```python
from build123d import *

# Parameters (mm, degrees)
SKETCH4_R          = 0.5
CUT_EXTRUDE1_DEPTH = 24.108440155
SKETCH5_R          = 2.5
CUT_EXTRUDE2_DEPTH = 2


with BuildPart() as part:
    # Loft1: read off the stored shape, not the designer's step
    # Loft1: loft between two sections, ruled curve by curve
    loft1_from = [
        Edge.make_bspline([(4.934796286, 0, 0.8048513), (3.325093686, 0, 10.674443872), (-6.544498886, 0, 9.064741272), (-4.934796286, 0, -0.8048513), (-3.325093686, 0, -10.674443872), (6.544498886, 0, -9.064741272), (4.934796286, 0, 0.8048513)], [0, 0, 0, 0, 0.5, 0.5, 0.5, 1, 1, 1, 1], 3, [1, 0.333333333, 0.333333333, 1, 0.333333333, 0.333333333, 1]),
    ]
    loft1_to = [
        Edge.make_bspline([(2.155997578, -22, 3.949895498), (-5.743793417, -22, 8.261890654), (-10.055788574, -22, 0.362099658), (-2.155997578, -22, -3.949895498), (5.743793417, -22, -8.261890654), (10.055788574, -22, -0.362099658), (2.155997578, -22, 3.949895498)], [0, 0, 0, 0, 0.5, 0.5, 0.5, 1, 1, 1, 1], 3, [1, 0.333333333, 0.333333333, 1, 0.333333333, 0.333333333, 1]),
    ]
    loft1 = Solid(Shell([*[Face.make_surface_from_curves(loft1_from[k], loft1_to[k]) for k in range(1)], Face(Wire(loft1_from)), Face(Wire(loft1_to))]))
    add(loft1)

    # Sketch4 → Cut-Extrude1 (cut, through all)
    with BuildSketch(Plane(origin=(0, 0, 0), x_dir=(1, 0, 0), z_dir=(0, 1, 0))):
        with Locations(Location((0, 0, 0), (0, 0, 270))):
            Circle(SKETCH4_R)
    extrude(amount=-CUT_EXTRUDE1_DEPTH, mode=Mode.SUBTRACT)

    # Sketch5 → Cut-Extrude2 (cut)
    with BuildSketch(Plane.XZ.offset(22)):
        with Locations(Location((0, 0, 0), (0, 0, 270))):
            Circle(SKETCH5_R)
    extrude(amount=-CUT_EXTRUDE2_DEPTH, mode=Mode.SUBTRACT)


solid = part.part
```
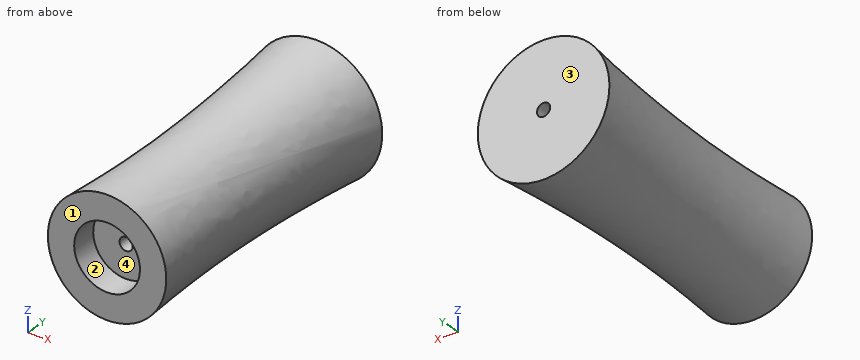
Input: part model. Units: mm. Frame: model coordinates. Face numbers are marked on the shaded views. A direction names the side the tool comes from. Give positions to 0.01 mm unless a question says otherwise; leave off trailing zeros. Answer as CSV lines item,"result". Start each with the question number.
1. Pull-direction query (Z, two-part tool) for the marked faces 3 and 4; classes: released by +Z, released by -Z, zero draft, split by the parting line, or undercut.
2. Pin query (flat end, axial travel): P1, Ø5, axis at x = -4, y = -12, coming from the +Z side; P2, Ø6, axis at x = 0, y = -10.5, coming from the -Z side; P3, Ø5, axis at y = -7, z = 2, coming from the -X side. Return the tip coordinate at first contact, or that it passes through.
3. Reachability of the marked faces 1 and 2 from +Z, -Z, +X, -X, +Y, -Y: full face, straight path, thin tool, end or side. Return the list, or none.
4. Line query: L1, parallel to X at y = -21.3, z = 0; L2, parallel to X at y = -12.25, z = 0; L3, parallel to Y at x = 1, z = 0.75. Output: solid intervals per line, ascending.
Computed values:
1,face 3,"zero draft"
1,face 4,"undercut"
2,P1,"stops at z = 3.98"
2,P2,"stops at z = -4.41"
2,P3,"stops at x = -4.54"
3,face 1,"+Z, -Z, +X, -X, -Y"
3,face 2,"-Y"
4,L1,"x = -4.46 to -2.5, 2.5 to 4.46"
4,L2,"x = -4.24 to -0.5, 0.5 to 4.24"
4,L3,"y = -20 to 0"
